Source: CAD feature listing. Evaluate the final solid. Frame: model axes, mm. A direction names the side the tool comes from. Coordinates: 2 decimals unless noted, no trailing zeros. Loops run counter-clockwise (first coordinate to the right, second up) from the corner with the lowest first, then second, coordinate; pieces in that order, holes last. Notation, with made-up numbers: (77.25, 36) -> (94.25, 36) arc R18 ccw to (94.25, 67) -> close; hole circle Ø10 at (6.25, 68). An arc over 180 degrees is marked (long way). Answer as a JSON object with one key per item and string values. Group by question number.
from build123d import *

# Parameters (mm, degrees)
SKETCH1_W               = 200
SKETCH1_H               = 200
BOSS_EXTRUDE1_DEPTH     = 1000
CUT_EXTRUDE1_DEPTH      = 100
CUT_EXTRUDE1_DEPTH_BACK = 300
SKETCH2_R               = 70
SKETCH3_W               = 100
SKETCH3_H               = 100
BOSS_EXTRUDE2_DEPTH     = 100
CUT_EXTRUDE2_DEPTH      = 20
CUT_EXTRUDE2_DEPTH_BACK = 130
SKETCH4_R               = 25
SKETCH7_R               = 50
CUT_EXTRUDE5_DEPTH      = 40
CUT_EXTRUDE6_START      = -40
SKETCH6_R               = 50
CUT_EXTRUDE6_DEPTH      = 40


with BuildPart() as part:
    # Sketch1 → Boss-Extrude1 (new body)
    with BuildSketch(Plane.XY):
        Rectangle(SKETCH1_W, SKETCH1_H)
    extrude(amount=BOSS_EXTRUDE1_DEPTH)

    # Sketch2 → Cut-Extrude1 (cut, two sides: drawn at the far end of the back side and taken through both)
    with BuildSketch(Plane(origin=(100, 0, 0), x_dir=(0, 0, -1), z_dir=(1, 0, 0)).offset(-CUT_EXTRUDE1_DEPTH_BACK)):
        with Locations(Location((-100, 0, 0), (0, 0, 180))):
            Circle(SKETCH2_R)
    extrude(amount=CUT_EXTRUDE1_DEPTH + CUT_EXTRUDE1_DEPTH_BACK, mode=Mode.SUBTRACT)

    # Sketch3 → Boss-Extrude2 (add)
    with BuildSketch(Plane.XY.offset(1000)):
        Rectangle(SKETCH3_W, SKETCH3_H)
    extrude(amount=BOSS_EXTRUDE2_DEPTH)

    # Sketch4 → Cut-Extrude2 (cut, two sides: drawn at the far end of the back side and taken through both)
    with BuildSketch(Plane(origin=(0, -50, 0), x_dir=(-1, 0, 0), z_dir=(0, -1, 0)).offset(-CUT_EXTRUDE2_DEPTH_BACK)):
        with Locations((0, -1050)):
            Circle(SKETCH4_R)
    extrude(amount=CUT_EXTRUDE2_DEPTH + CUT_EXTRUDE2_DEPTH_BACK, mode=Mode.SUBTRACT)

    # Sketch7 → Cut-Extrude5 (cut)
    with BuildSketch(Plane.ZY.offset(100)):
        with Locations((750, 0)):
            Circle(SKETCH7_R)
    extrude(amount=-CUT_EXTRUDE5_DEPTH, mode=Mode.SUBTRACT)

    # Sketch6 → Cut-Extrude6 (cut)
    with BuildSketch(Plane(origin=(100, 0, 0), x_dir=(0, 0, -1), z_dir=(1, 0, 0)).offset(CUT_EXTRUDE6_START)):
        with Locations(Location((-750, 0, 0), (0, 0, 180))):
            Circle(SKETCH6_R)
    extrude(amount=CUT_EXTRUDE6_DEPTH, mode=Mode.SUBTRACT)


solid = part.part
1. Section query A-A on y = 0. Return loops of the section in (x, z), then the cut area to 3 significant figures.
2. Section query B-B on z = 100. Return loops of the section in (x, y).
3. Section query D-D on z = 750. Return loops of the section in (x, y).
4. Ray query, L1, parallel to Z at x = 90, y = 1; L2, parallel to X at y = 25, z = 1050; L3, parallel to Y at x = -85, z = 750. Return the intervals inside material, ascending.
5. Section query C-C on x = 0. Return loops of the section in (y, z), then the cut area to 3 significant figures.
6. Reachability of faces 1 (the face through (-50, -1, 1049)), 2 (the face through (-80.28, 15.02, 797.69)), 3 (the face through (60, -1, 749)), 4 (the face through (50, -1, 1049)) from +Z, -Z, +X, -X, +Y, -Y: full face, straight path, thin tool, end or side. Return the list, or none.
7. Mould query, pull axis Y, two halves, no side actions, for faces 5 (the face through (-12, 50, 1027)), 6 (the face through (-68, 1, 1000)), 7 (the face through (79.72, -15.02, 797.69)), 8 (the face through (-12, -50, 1027)). Classes: pulls with the +Y half, pulls with the -Y half, needs draft (parallel to the pull), parting line crosses it, or undercut.
Solved:
{
 "1": {"outline": "(-100, 0) -> (100, 0) -> (100, 30) -> (-100, 30) -> close; (-100, 170) -> (100, 170) -> (100, 700) -> (60, 700) -> (60, 800) -> (100, 800) -> (100, 1000) -> (50, 1000) -> (50, 1100) -> (-50, 1100) -> (-50, 1000) -> (-100, 1000) -> (-100, 800) -> (-60, 800) -> (-60, 700) -> (-100, 700) -> close; hole circle Ø50 at (0, 1050)", "area": "172,000 mm^2"},
 "2": {"outline": "(-100, -100) -> (100, -100) -> (100, -70) -> (-100, -70) -> close; (-100, 70) -> (100, 70) -> (100, 100) -> (-100, 100) -> close"},
 "3": {"outline": "(-100, -100) -> (100, -100) -> (100, -50) -> (60, -50) -> (60, 50) -> (100, 50) -> (100, 100) -> (-100, 100) -> (-100, 50) -> (-60, 50) -> (-60, -50) -> (-100, -50) -> close"},
 "4": {"L1": "0 to 30.01, 169.99 to 700.01, 799.99 to 1000", "L2": "-50 to -25, 25 to 50", "L3": "-100 to -50, 50 to 100"},
 "5": {"outline": "(-100, 0) -> (100, 0) -> (100, 1000) -> (50, 1000) -> (50, 1025) -> (-50, 1025) -> (-50, 1000) -> (-100, 1000) -> close; (-50, 1075) -> (50, 1075) -> (50, 1100) -> (-50, 1100) -> close; hole circle Ø140 at (0, 100)", "area": "190,000 mm^2"},
 "6": {"face 1": "+Z, -X, +Y, -Y", "face 2": "-X", "face 3": "+X", "face 4": "+Z, +X, +Y, -Y"},
 "7": {"face 5": "pulls with the +Y half", "face 6": "needs draft", "face 7": "undercut", "face 8": "pulls with the -Y half"}
}
